Could you check a few things on this model? Use its own coordinates, in mm. A direction names the side the tool comes from. Coordinates: 2 decimals unless noted, no trailing zeros. Order: outer loops, then holes, each group sorted by start corner. A loop starts at its lowest first (then second) coordinate and runs counter-clockwise, first axis right, second up. Notation, with made-up numbers: (30, 3.25) - (39, 3.25) arc R16 ccw to (39, 30.25) - close; hole circle Ø7 at (89.5, 66.25). An arc over 180 degrees is marked (long way). One line per item, written item: value.
from build123d import *

# Parameters (mm, degrees)
SKETCH1_W                       = 106
SKETCH1_H                       = 68
BOSS_EXTRUDE1_DEPTH             = 0.6
SKETCH2_W                       = 95
SKETCH2_H                       = 54.6
CUT_EXTRUDE1_DEPTH              = 0.1
SKETCH4_W                       = 104.2
SKETCH4_H                       = 66.2
BOSS_EXTRUDE2_DEPTH             = 4
SKETCH5_W                       = 102
SKETCH5_H                       = 64
BOSS_EXTRUDE3_DEPTH             = 2.4
SKETCH6_W                       = 106.4
SKETCH6_H                       = 68.5
BOSS_EXTRUDE4_DEPTH             = 1.6
BOSS_EXTRUDE5_DEPTH             = 2.8
BOSS_EXTRUDE5_DIRECTION_2_REACH = 88.689
FILLET1_R                       = 2
CUT_EXTRUDE2_REACH              = 114.578
SKETCH9_R                       = 2.75
BOSS_EXTRUDE6_DEPTH             = 4.5
SKETCH10_R                      = 1.25
CUT_EXTRUDE3_DEPTH              = 6.1
SKETCH11_W                      = 2.5
SKETCH11_H                      = 22
BOSS_EXTRUDE7_DEPTH             = 5.6
SKETCH12_W                      = 23.5
SKETCH12_H                      = 6
SKETCH12_W_2                    = 6.5
BOSS_EXTRUDE8_DEPTH             = 3


with BuildPart() as part:
    # Sketch1 → Boss-Extrude1 (new body)
    with BuildSketch(Plane.XY):
        Rectangle(SKETCH1_W, SKETCH1_H)
    extrude(amount=BOSS_EXTRUDE1_DEPTH)

    # Sketch2 → Cut-Extrude1 (cut)
    with BuildSketch(Plane.XY.offset(0.6)):
        with Locations((0, 2.3)):
            Rectangle(SKETCH2_W, SKETCH2_H)
    extrude(amount=-CUT_EXTRUDE1_DEPTH, mode=Mode.SUBTRACT)

    # Sketch4 → Boss-Extrude2 (add)
    with BuildSketch(Plane(origin=(0, 0, 0), x_dir=(-1, 0, 0), z_dir=(0, 0, -1))):
        Rectangle(SKETCH4_W, SKETCH4_H)
    extrude(amount=BOSS_EXTRUDE2_DEPTH)

    # Sketch5 → Boss-Extrude3 (add)
    with BuildSketch(Plane(origin=(0, 0, -4), x_dir=(-1, 0, 0), z_dir=(0, 0, -1))):
        Rectangle(SKETCH5_W, SKETCH5_H)
    extrude(amount=BOSS_EXTRUDE3_DEPTH)

    # Sketch6 → Boss-Extrude4 (add)
    with BuildSketch(Plane(origin=(0, 0, -6.4), x_dir=(-1, 0, 0), z_dir=(0, 0, -1))):
        with Locations((1.1, -1.05)):
            Rectangle(SKETCH6_W, SKETCH6_H)
    extrude(amount=BOSS_EXTRUDE4_DEPTH)

    # Sketch7 → Boss-Extrude5 (add)
    with BuildSketch(Plane.XZ.offset(33.1)):
        Polygon((47.5, 0), (42.5, -5), (28.5, -5), (23.5, 0), align=None)
    extrude(amount=BOSS_EXTRUDE5_DEPTH)

    # Boss-Extrude5 direction 2: up to this face of the body (flat: up to its plane)
    boss_extrude5_direction_2_end = Plane(part.part.faces().sort_by_distance((0, -32, -5.2))[0])
    # Sketch7 → Boss-Extrude5 direction 2 (add, up to the picked face)
    with BuildSketch(Plane.XZ.offset(33.1), mode=Mode.PRIVATE) as boss_extrude5_direction_2_sk1:
        Polygon((47.5, 0), (42.5, -5), (28.5, -5), (23.5, 0), align=None)
    boss_extrude5_direction_2_tool1 = split(extrude(boss_extrude5_direction_2_sk1.sketch, amount=-BOSS_EXTRUDE5_DIRECTION_2_REACH, mode=Mode.PRIVATE), bisect_by=boss_extrude5_direction_2_end, keep=Keep.BOTH, mode=Mode.PRIVATE)
    add(boss_extrude5_direction_2_tool1.solids().sort_by(Axis((35.5, -33.1, -2.280702), (0, 1, 0)))[0])

    # Fillet1
    # the kernel refuses this fillet: 2 mm, written as the material it takes off along each edge
    with BuildSketch(Plane(origin=(18.506253911, -35.9, 0), x_dir=(0, 1, 0), z_dir=(1, 0, 0))) as fillet1_piece_1:
        with BuildLine():
            CenterArc((2, -1.997498436), FILLET1_R, 92.865983983, 87.134016017)
            Line((0, -1.997498436), (-0.04, -1.997498436))
            Line((-0.04, -1.997498436), (-0.04, 0))
            Line((-0.04, 0), (0, 0.04))
            ThreePointArc((0, 0.04), (0.95, 0.04), (1.898, 0.039949969))
            Line((1.898, 0.039949969), (1.9, 0))
        make_face()
    extrude(amount=33.987492178, mode=Mode.SUBTRACT)
    with BuildSketch(Plane(origin=(47.5, -35.9, -5), x_dir=(0, 0, 1), z_dir=(-1, 0, 0))) as fillet1_piece_2:
        with BuildLine():
            CenterArc((FILLET1_R, FILLET1_R), FILLET1_R, 180, 90)
            Line((0, FILLET1_R), (-FILLET1_R * 0.02, FILLET1_R))
            Line((-FILLET1_R * 0.02, FILLET1_R), (-FILLET1_R * 0.02, -FILLET1_R * 0.02))
            Line((-FILLET1_R * 0.02, -FILLET1_R * 0.02), (FILLET1_R, -FILLET1_R * 0.02))
            Line((FILLET1_R, -FILLET1_R * 0.02), (FILLET1_R, 0))
        make_face()
    extrude(amount=24, mode=Mode.SUBTRACT)

    # Cut-Extrude2: up to this plane
    cut_extrude2_end = Plane(origin=(28.5, -7.484698656, -5), z_dir=(-0.7071067811865419, 0, -0.7071067811865531))
    # Sketch8 → Cut-Extrude2 (cut, up to the surface)
    with BuildSketch(Plane(origin=(52.1, 0, 0), x_dir=(0, 0, -1), z_dir=(1, 0, 0)), mode=Mode.PRIVATE) as cut_extrude2_sk1:
        with BuildLine():
            Line((4.825635078, -32.015779283), (4, -32.015779283))
            Line((4, -32.015779283), (4, -33.1))
            Line((4, -33.1), (0.255629625, -33.1))
            add(Edge.make_bspline(
                [(0.255629625, -33.1), (-0.100580752, -35.335403533), (4.586512434, -36.596617464), (4.967609775, -32.916750312), (4.825635078, -32.015779283)],
                knots=[0, 0, 0, 0, 0.609319743, 1, 1, 1, 1], degree=3))
        make_face()
    cut_extrude2_tool1 = split(extrude(cut_extrude2_sk1.sketch, amount=-CUT_EXTRUDE2_REACH, mode=Mode.PRIVATE), bisect_by=cut_extrude2_end, keep=Keep.BOTH, mode=Mode.PRIVATE)
    add(cut_extrude2_tool1.solids().sort_by_distance((52.1, -33.994656, -2.685344))[0], mode=Mode.SUBTRACT)

    # Sketch9 → Boss-Extrude6 (add)
    with BuildSketch(Plane(origin=(0, 0, -8), x_dir=(-1, 0, 0), z_dir=(0, 0, -1))):
        with Locations((-48.55, 29.85)):
            Circle(SKETCH9_R)
        with Locations((-48.55, -31.95)):
            Circle(SKETCH9_R)
        with Locations((50.75, 29.85)):
            Circle(SKETCH9_R)
        with Locations((50.75, -31.95)):
            Circle(SKETCH9_R)
        with Locations((-26.25, 23.6)):
            Circle(SKETCH9_R)
        with Locations((-26.25, -25.7)):
            Circle(SKETCH9_R)
        with Locations((31.65, 23.6)):
            Circle(SKETCH9_R)
        with Locations((31.65, -25.7)):
            Circle(SKETCH9_R)
    extrude(amount=BOSS_EXTRUDE6_DEPTH)

    # Sketch10 → Cut-Extrude3 (cut)
    with BuildSketch(Plane(origin=(0, 0, -12.5), x_dir=(-1, 0, 0), z_dir=(0, 0, -1))):
        with Locations((-48.55, 29.85)):
            Circle(SKETCH10_R)
        with Locations((-26.25, 23.6)):
            Circle(SKETCH10_R)
        with Locations((31.65, 23.6)):
            Circle(SKETCH10_R)
        with Locations((50.75, 29.85)):
            Circle(SKETCH10_R)
        with Locations((-26.25, -25.7)):
            Circle(SKETCH10_R)
        with Locations((-48.55, -31.95)):
            Circle(SKETCH10_R)
        with Locations((50.75, -31.95)):
            Circle(SKETCH10_R)
        with Locations((31.65, -25.7)):
            Circle(SKETCH10_R)
    extrude(amount=-CUT_EXTRUDE3_DEPTH, mode=Mode.SUBTRACT)

    # Sketch11 → Boss-Extrude7 (add)
    with BuildSketch(Plane(origin=(0, 0, -8), x_dir=(-1, 0, 0), z_dir=(0, 0, -1))):
        with Locations((50.75, -1.05)):
            Rectangle(SKETCH11_W, SKETCH11_H)
    extrude(amount=BOSS_EXTRUDE7_DEPTH)

    # Sketch12 → Boss-Extrude8 (add)
    with BuildSketch(Plane(origin=(0, 0, -8), x_dir=(-1, 0, 0), z_dir=(0, 0, -1))):
        with Locations((25.15, 7.4)):
            Rectangle(SKETCH12_W, SKETCH12_H)
        with Locations((-32.65, -12.3)):
            Rectangle(SKETCH12_W_2, SKETCH12_H)
    extrude(amount=BOSS_EXTRUDE8_DEPTH)


solid = part.part
Item 1: For faces 4 (the face through (-48.003, 29.971, -10.218)), 5 (the face through (33, -12, -11)), 6 (the face through (1, 33.1, -2)), 7 (the face through (-52, -1, -11)), which set-ups out of +Z, -Z, +X, -X, +Y, -Y let a thin tool reach every point of the face, with its end or its side?
Conclusion:
face 4: -Z
face 5: -Z, +X, +Y, -Y
face 6: +X, -X, +Y
face 7: -Z, -X
Item 2: I want a section at C-C on y = 6.5. Please give me the cut outline in (x, z).
Conclusion:
outline: (-54.3, -8) - (-52, -8) - (-52, -13.6) - (-49.5, -13.6) - (-49.5, -8) - (-36.9, -8) - (-36.9, -11) - (-13.4, -11) - (-13.4, -8) - (52.1, -8) - (52.1, -6.4) - (51, -6.4) - (51, -4) - (52.1, -4) - (52.1, 0) - (53, 0) - (53, 0.6) - (47.5, 0.6) - (47.5, 0.5) - (-47.5, 0.5) - (-47.5, 0.6) - (-53, 0.6) - (-53, 0) - (-52.1, 0) - (-52.1, -4) - (-51, -4) - (-51, -6.4) - (-54.3, -6.4) - close
Item 3: I want a section at A-A on z = -9.25. Give the number of separate pieces and of enclosed holes in the cut face, then the cut area to 3 significant figures.
Conclusion:
separate pieces: 11
enclosed holes: 8
area: 386 mm²
Item 4: I'm going to push flat-ended pins straight in: pin 1 Ø8 at (x, y) = (37.5, -10.5) entering from -Z; pin 2 Ø1 at (x, y) = (-50.5, -31.5) entering from -Z; pin 3 Ø3.5 at (y, z) = (8, -9) entering from +X. Where does each tip first touch, or does it pass through?
Conclusion:
pin 1: z = -11
pin 2: z = -6.4
pin 3: x = 52.1
Item 5: If I drill on probe 1 along Y at (x, z) = (48.55, -9.5); probe 2 along Y at (x, z) = (-31.65, -10.75); probe 3 along Z at (x, y) = (-45, -26), over which ranges is the centre line in solid material (lowest first)?
Conclusion:
probe 1: -34.7 to -33.2, -30.7 to -29.2, 27.1 to 28.6, 31.1 to 32.6
probe 2: -28.45 to -26.95, -24.45 to -22.95, 4.4 to 10.4, 20.85 to 22.35, 24.85 to 26.35
probe 3: -8 to 0.6
Item 6: I want a section at D-D on x = -43. Please give me the cut outline in (y, z), then the cut area to 3 significant figures.
Conclusion:
outline: (-35.3, -8) - (33.2, -8) - (33.2, -6.4) - (32, -6.4) - (32, -4) - (33.1, -4) - (33.1, 0) - (34, 0) - (34, 0.6) - (29.6, 0.6) - (29.6, 0.5) - (-25, 0.5) - (-25, 0.6) - (-34, 0.6) - (-34, 0) - (-33.1, 0) - (-33.1, -4) - (-32, -4) - (-32, -6.4) - (-35.3, -6.4) - close
area: 563 mm²
Item 7: Thinking about a two-plate mould opening in Z: for faces 1 (the face through (-4, -28, 0.6)), 2 (the face through (35.63, -35.3, -4.43)), 3 (the face through (-49.5, -1, -11)), which applies, pulls with the +Z half, pulls with the -Z half, needs draft (parallel to the pull), parting line crosses it, or undercut?
Conclusion:
face 1: pulls with the +Z half
face 2: undercut
face 3: needs draft
